```python
from build123d import *

# Parameters (mm, degrees)
SKETCH2_W               = 88.9
SKETCH2_H               = 152.4
BOSS_EXTRUDE1_DEPTH     = 5.9944
SKETCH4_R               = 2.7305
CUT_EXTRUDE2_DEPTH      = 1
CUT_EXTRUDE2_DEPTH_BACK = 6.9944
SKETCH5_R               = 2.7305
CUT_EXTRUDE3_DEPTH      = 1
CUT_EXTRUDE3_DEPTH_BACK = 6.9944
SKETCH6_R               = 1.905
CUT_EXTRUDE4_DEPTH      = 1
CUT_EXTRUDE4_DEPTH_BACK = 6.9944
SKETCH7_W               = 2.54
SKETCH7_H               = 152.4
CUT_EXTRUDE5_DEPTH      = 1
CUT_EXTRUDE5_DEPTH_BACK = 6.9944


with BuildPart() as part:
    # Sketch2 → Boss-Extrude1 (new body)
    with BuildSketch(Plane(origin=(0, 0, 0), x_dir=(1, 0, 0), z_dir=(0, 1, 0))):
        with Locations((44.45, 76.2)):
            Rectangle(SKETCH2_W, SKETCH2_H)
    extrude(amount=BOSS_EXTRUDE1_DEPTH)

    # Sketch4 → Cut-Extrude2 (cut, two sides)
    with BuildSketch(Plane(origin=(0, 5.9944, 0), x_dir=(1, 0, 0), z_dir=(0, 1, 0))) as cut_extrude2_sk:
        with Locations((45.72, 100.33)):
            Circle(SKETCH4_R)
        with Locations((45.72, 24.13)):
            Circle(SKETCH4_R)
    extrude(amount=CUT_EXTRUDE2_DEPTH, mode=Mode.SUBTRACT)
    extrude(cut_extrude2_sk.sketch, amount=-CUT_EXTRUDE2_DEPTH_BACK, mode=Mode.SUBTRACT)

    # Sketch5 → Cut-Extrude3 (cut, two sides)
    with BuildSketch(Plane(origin=(0, 5.9944, 0), x_dir=(1, 0, 0), z_dir=(0, 1, 0))) as cut_extrude3_sk:
        with Locations((50.8, 63.5)):
            Circle(SKETCH5_R)
        with Locations((50.8, 12.7)):
            Circle(SKETCH5_R)
    extrude(amount=CUT_EXTRUDE3_DEPTH, mode=Mode.SUBTRACT)
    extrude(cut_extrude3_sk.sketch, amount=-CUT_EXTRUDE3_DEPTH_BACK, mode=Mode.SUBTRACT)

    # Sketch6 → Cut-Extrude4 (cut, two sides)
    with BuildSketch(Plane(origin=(0, 5.9944, 0), x_dir=(1, 0, 0), z_dir=(0, 1, 0))) as cut_extrude4_sk:
        with Locations((45.6438, 109.2962)):
            Circle(SKETCH6_R)
        with Locations((8.89, 109.2962)):
            Circle(SKETCH6_R)
        with Locations((8.89, 146.05)):
            Circle(SKETCH6_R)
        with Locations((45.6438, 146.05)):
            Circle(SKETCH6_R)
    extrude(amount=CUT_EXTRUDE4_DEPTH, mode=Mode.SUBTRACT)
    extrude(cut_extrude4_sk.sketch, amount=-CUT_EXTRUDE4_DEPTH_BACK, mode=Mode.SUBTRACT)

    # Sketch7 → Cut-Extrude5 (cut, two sides)
    with BuildSketch(Plane(origin=(0, 5.9944, 0), x_dir=(1, 0, 0), z_dir=(0, 1, 0))) as cut_extrude5_sk:
        with Locations((1.27, 76.2)):
            Rectangle(SKETCH7_W, SKETCH7_H)
    extrude(amount=CUT_EXTRUDE5_DEPTH, mode=Mode.SUBTRACT)
    extrude(cut_extrude5_sk.sketch, amount=-CUT_EXTRUDE5_DEPTH_BACK, mode=Mode.SUBTRACT)


solid = part.part
```
CAD build for the part. Positions are in the model's coordinates, mm. Round coordinates to 2 decimals unless told otherwise and drop trailing zeros. Order: outer loops, then holes, each group sorted by start corner. A loop starts at its lowest first (then second) coordinate and runs counter-clockwise, first axis right, second up.
Q1. Two-plate mould, pull along Z, no slides. Class faces 1 (the cylindrical face through (8.642, 3.039, -111.185)), 2 (the flat face through (45, 0, -77)), 3 (the flat face through (45, 3, -152.4)): pulls with the +Z half, pulls with the -Z half, needs draft (parallel to the pull), parting line crosses it, or undercut.
Q2. Slice it at A-A (x = 50.8). Write the cut outline in (y, z).
Q3. Slice it at B-B (z = -146.05). Write the cut outline in (x, y) (3 decimals).
Q4. Slice it at C-C (z = -100.33). Write the cut outline in (x, y), and give its area (3 significant figures).
Q5. Wall check: L1, parallel to Z at x = 8.89, y = 3.85 (3 decimals); L2, parallel to Z at x = 50.8, y = 2.75; L3, parallel to X at y = 2.4, z = -146.05 (3 decimals). Give the ranges that are in metal, low to high.
Results below:
1. face 1: undercut
1. face 2: needs draft
1. face 3: pulls with the -Z half
2. outline: (0, -152.4) - (5.99, -152.4) - (5.99, -66.23) - (0, -66.23) - close; (0, -60.77) - (5.99, -60.77) - (5.99, -15.43) - (0, -15.43) - close; (0, -9.97) - (5.99, -9.97) - (5.99, 0) - (0, 0) - close
3. outline: (2.54, 0) - (6.985, 0) - (6.985, 5.994) - (2.54, 5.994) - close; (10.795, 0) - (43.739, 0) - (43.739, 5.994) - (10.795, 5.994) - close; (47.549, 0) - (88.9, 0) - (88.9, 5.994) - (47.549, 5.994) - close
4. outline: (2.54, 0) - (42.99, 0) - (42.99, 5.99) - (2.54, 5.99) - close; (48.45, 0) - (88.9, 0) - (88.9, 5.99) - (48.45, 5.99) - close
4. area: 485 mm2
5. L1: z = -152.4 to -147.955, -144.145 to -111.201, -107.391 to 0
5. L2: z = -152.4 to -66.23, -60.77 to -15.43, -9.97 to 0
5. L3: x = 2.54 to 6.985, 10.795 to 43.739, 47.549 to 88.9
